Work out the finished part from the listing and answer in its coordinate system (mm). Face numbers are marked on the shaded views. Give positions to 0.01 mm unless a question says otherwise; leave off trailing zeros. Loops run counter-clockwise (first coordinate to the right, second up) from the corner with the lowest first, then second, coordinate; pieces in that order, holes last. Notation, with made-up numbers: M 51,-26 L 85,-26 A21 ccw 85,-12 Z; hole C 5.25,-16.5 d3. An arc over 180 degrees is marked long. Use a Markdown table: item, result.
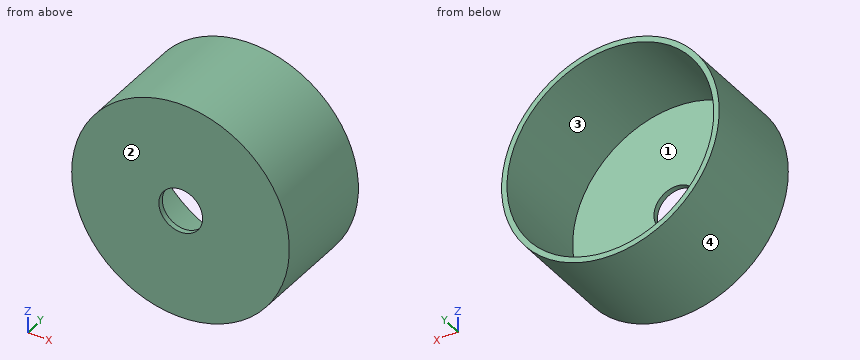
Autodesk Inventor part; units mm, degrees
ref_plane "YZ Plane" through (0, 0, 0) normal (1, 0, 0) x (0, 1, 0)
ref_plane "XZ Plane" through (0, 0, 0) normal (0, 1, 0) x (-1, 0, 0)
ref_plane "XY Plane" through (0, 0, 0) normal (0, 0, 1) x (1, 0, 0)
sketch "Boceto1" plane through (0, 0, 0) normal (0, 1, 0) x (-1, 0, 0)
  circle A0 centre (0, 0) radius 100
  dimension "d0" = 200
extrude "Extrusión1" add sketch "Boceto1" along normal mid plane 100
shell "Vaciado1" thickness 5 removed faces 1 at (-44.3571, 50, 16.5389)
sketch "Boceto2" plane through (0, -50, 0) normal (0, -1, 0) x (1, 0, 0)
  point P0 (0, 0)
  point P1 (0.1915, 0)
hole "Agujero1" at (0.1915, -50, 0) direction (0, 1, 0) diameter 40.241 end through all
properties part number "base redonda"
(1) Consider probe 1 along Z at (x, y) = (0, 12); probe 2 along X at (y, z) = (28, -1) (3 decimals); probe 3 along Y at (x, z) = (53.5, 12.5). Determine where each line is inside the solid, lowest interval first. Write a range as [from, to].
Entries:
| item | result |
|---|---|
| probe 1 | z = [-100, -95], [95, 100] |
| probe 2 | x = [-99.995, -94.995], [94.995, 99.995] |
| probe 3 | y = [-50, -45] |
(2) A cutting plane is placed at C-C (y = -25.5). Write down the section's boundary in (x, z), and give its area (3 significant figures).
Entries:
| item | result |
|---|---|
| outline | C 0,0 d200; hole C 0,0 d190 |
| area | 3,060 mm² |
(3) A cutting plane is placed at A-A (z = 0). Write down the section's boundary in (x, y), and give its area (3 significant figures).
Entries:
| item | result |
|---|---|
| outline | M -100,-50 L -19.93,-50 L -19.93,-45 L -95,-45 L -95,50 L -100,50 Z; M 20.31,-50 L 100,-50 L 100,50 L 95,50 L 95,-45 L 20.31,-45 Z |
| area | 1,750 mm² |
(4) The mould has two halves that part along X. Classify the marked faces 1, 2, 3 and 4: released by +X, released by -X, zero draft, split by the parting line, or undercut.
Entries:
| item | result |
|---|---|
| face 1 | undercut |
| face 2 | zero draft |
| face 3 | undercut |
| face 4 | split by the parting line |
(5) Given P1, Ø1, axis at y = -36.5, z = 19.5, coming from the -X side; P2, Ø1, axis at y = -31, z = -8.5, coming from the +X side; P3, Ø4, axis at y = 8.5, z = 37.5, coming from the -X side, each flat-ended and moving along its own axis, determine where each tip first touches the part or whether it passes through.
Entries:
| item | result |
|---|---|
| P1 | stops at x = -98.18 |
| P2 | stops at x = 99.68 |
| P3 | stops at x = -93.49 |
(6) A cutting plane is placed at D-D (z = 77). Write down the section's boundary in (x, y).
Entries:
| item | result |
|---|---|
| outline | M -63.8,-50 L 63.8,-50 L 63.8,50 L 55.64,50 L 55.64,-45 L -55.64,-45 L -55.64,50 L -63.8,50 Z |
(7) A cutting plane is placed at B-B (x = -6). Write down the section's boundary in (y, z).
Entries:
| item | result |
|---|---|
| outline | M -50,-99.82 L 50,-99.82 L 50,-94.81 L -45,-94.81 L -45,-19.14 L -50,-19.14 Z; M -50,19.14 L -45,19.14 L -45,94.81 L 50,94.81 L 50,99.82 L -50,99.82 Z |
